Read the model definition and answer for the solid it produces. Units are mm, in the model's axes. Face numbers are marked on the shaded views. A direction names the side the tool comes from. Give positions to 0.01 mm unless a question says otherwise; leave off trailing zeros. Order: outer loops, then holes, each group sorted by start corner. A loop starts at its lowest first (then second) coordinate and runs counter-clockwise, first axis right, second up. Notation, with made-up numbers: (-1.75, 79) - (28.25, 79) arc R6 cw to (28.25, 83) - close; hole circle Ø5 at (1.25, -25.75). An arc over 180 degrees is marked (long way). Write item = value, one per line.
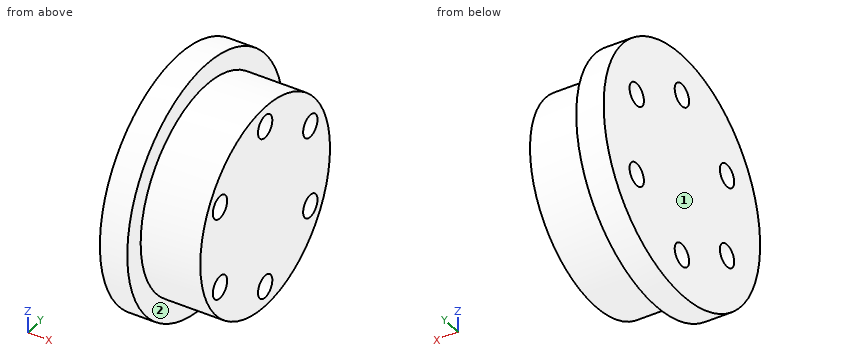
```python
from build123d import *

# Parameters (mm, degrees)
SKETCH1_R           = 18
BOSS_EXTRUDE1_DEPTH = 4
SKETCH2_R           = 14.925
BOSS_EXTRUDE2_DEPTH = 8.7
SKETCH3_R           = 1.65
CUT_EXTRUDE1_DEPTH  = 29.448022778


with BuildPart() as part:
    # Sketch1 → Boss-Extrude1 (new body)
    with BuildSketch(Plane.YZ):
        with Locations(Location((0, 0, 0), (0, 0, 270))):
            Circle(SKETCH1_R)
    extrude(amount=BOSS_EXTRUDE1_DEPTH)

    # Sketch2 → Boss-Extrude2 (add)
    with BuildSketch(Plane.YZ.offset(4)):
        with Locations(Location((0, 0, 0), (0, 0, 270))):
            Circle(SKETCH2_R)
    extrude(amount=BOSS_EXTRUDE2_DEPTH)

    # Sketch3 → Cut-Extrude1 (cut, through all)
    with BuildSketch(Plane.YZ.offset(12.7)):
        with Locations(Location((0, 12, 0), (0, 0, 270))):
            Circle(SKETCH3_R)
        with Locations(Location((10.392304845, 6, 0), (0, 0, 270))):
            Circle(SKETCH3_R)
        with Locations(Location((10.392304845, -6, 0), (0, 0, 270))):
            Circle(SKETCH3_R)
        with Locations(Location((0, -12, 0), (0, 0, 270))):
            Circle(SKETCH3_R)
        with Locations(Location((-10.392304845, -6, 0), (0, 0, 270))):
            Circle(SKETCH3_R)
        with Locations(Location((-10.392304845, 6, 0), (0, 0, 270))):
            Circle(SKETCH3_R)
    extrude(amount=-CUT_EXTRUDE1_DEPTH, mode=Mode.SUBTRACT)


solid = part.part
```
1. Straight lines are drawn through the part: L1, parallel to Y at x = 10.25, z = -6; L2, parallel to Y at x = 8.5, z = -5.5; L3, parallel to X at y = -7, z = -15. For each, find the intervals that lie inside material, in ascending order. Write a range as [from, to].
Recorded:
L1 = [-13.67, -12.04], [-8.74, 8.74], [12.04, 13.67]
L2 = [-13.87, -11.96], [-8.82, 8.82], [11.96, 13.87]
L3 = [0, 4]
2. Section B-B (z = 12) is taken. Determine the outline of the cut face in (x, y).
Recorded:
outline = (0, -13.42) - (4, -13.42) - (4, -8.87) - (12.7, -8.87) - (12.7, -1.65) - (0, -1.65) - close; (0, 1.65) - (12.7, 1.65) - (12.7, 8.87) - (4, 8.87) - (4, 13.42) - (0, 13.42) - close
3. For the marked faces 1 and 2, determine the directions among +Z, -Z, +X, -X, +Y, -Y from which every point of the face is accessible in a straight line to the end or side of a thin tool.
Recorded:
face_1 = +Z, -Z, -X, +Y, -Y
face_2 = +X
4. Section A-A (y = 0) is taken. Determine the outline of the cut face in (x, z) (3 decimals), and give its area (3 significant figures).
Recorded:
outline = (0, -18) - (4, -18) - (4, -14.925) - (12.7, -14.925) - (12.7, -13.65) - (0, -13.65) - close; (0, -10.35) - (12.7, -10.35) - (12.7, 10.35) - (0, 10.35) - close; (0, 13.65) - (12.7, 13.65) - (12.7, 14.925) - (4, 14.925) - (4, 18) - (0, 18) - close
area = 320 mm^2
5. Flat-ended cylindrical pins translate along their axes: pin 1 (2 mm diameter, centred on x = 10, y = -6.5, fed in from +Z); pin 2 (6 mm diameter, centred on x = 6.5, z = -9.5, fed in from -Y); pin 3 (1 mm diameter, centred on x = 6, y = 3, fed in from +Z). Find the tip coordinate at first contact, or state that the pin passes through.
Recorded:
pin_1 = 13.87
pin_2 = -16.2
pin_3 = 14.71
6. Section C-C (z = 6) is taken. Determine the outline of the cut face in (x, y), and give its area (3 significant figures).
Recorded:
outline = (0, -16.97) - (4, -16.97) - (4, -13.67) - (12.7, -13.67) - (12.7, -12.04) - (0, -12.04) - close; (0, -8.74) - (12.7, -8.74) - (12.7, 8.74) - (0, 8.74) - close; (0, 12.04) - (12.7, 12.04) - (12.7, 13.67) - (4, 13.67) - (4, 16.97) - (0, 16.97) - close
area = 290 mm^2
7. Section D-D (y = -14) is taken. Determine the outline of the cut face in (x, z).
Recorded:
outline = (0, -11.31) - (4, -11.31) - (4, -5.17) - (12.7, -5.17) - (12.7, 5.17) - (4, 5.17) - (4, 11.31) - (0, 11.31) - close
